Here's how the part is built. I have some questions about the finished solid (model axes, mm). Coordinates: 2 decimals unless noted, no trailing zeros. Write each loop counter-clockwise with the first axis right and the second up, starting at its lowest first coordinate (ties: lowest second). Pieces come first, ordered by that corner, then holes.
Item 1: If we section it at A-A (x = 0): Please give me the cut outline in (y, z) (3 decimals), then the cut area to 3 significant figures.
Item 2: If we section it at B-B (y = -128): Please give me the cut outline in (x, z) (3 decimals).
Item 3: I'm going to push flat-ended pins straight in: pin 1 Ø4 at (y, z) = (-240, -18) entering from +X; pin 2 Ø11.5 at (x, z) = (0, 0) entering from +Y; pin 3 Ø1.5 at (y, z) = (-148, 9.5) entering from -X. Where does each tip first touch, or does it pass through?
Item 4: If I drill on line 1 (Y direction, x = -9, z = 13); line 2 (Z direction, x = 0, y = -126) (3 decimals), over which ranges is the centre line in solid material (lowest first)?
Item 5: If we section it at C-C (z = 0): Please give me the cut outline in (x, y) (3 decimals).
from build123d import *

# Parameters (mm, degrees)
F0_R          = 34.925
F0_R_2        = 28.575
F1_DEPTH      = 304.8
F2_R          = 34.925
F3_DEPTH      = 6.35
F4_R          = 34.925
F5_DEPTH      = 6.35
F6_R          = 6.35
F7_R          = 6.35
F8_W          = 228.6
F8_H          = 3.175
F10_S5_R      = 34.925
F10_T6_DEPTH  = 52
F10_S11_R     = 31.75
F10_T12_DEPTH = 51
F11_R         = 6.35
F12_DEPTH     = 25.4


# Not quite as in the source:
# - a fillet or chamfer that OpenCascade refuses, or shapes differently, is made with other operations: its cross-section is extruded or revolved along the edge and cut away or added


with BuildPart() as f1:
    # F0 (on Front) → F1 (new body)
    with BuildSketch(Plane.XZ):
        Circle(F0_R)
        Circle(F0_R_2, mode=Mode.SUBTRACT)
    extrude(amount=F1_DEPTH)

    # F2 (on face) → F3 (join)
    with BuildSketch(Plane.XZ.offset(304.8)):
        Circle(F2_R)
    extrude(amount=-F3_DEPTH)

    # F4 (on face) → F5 (join)
    with BuildSketch(Plane(origin=(0, 0, 0), x_dir=(-1, 0, 0), z_dir=(0, 1, 0))):
        Circle(F4_R)
    extrude(amount=-F5_DEPTH)

    # F6
    f6_edges = [f1.edges().sort_by_distance(p)[0] for p in [
        (-34.925, 0, 0),
    ]]
    fillet(f6_edges, radius=F6_R)

    # F7
    f7_edges = [f1.edges().sort_by_distance(p)[0] for p in [
        (-34.925, -304.8, 0),
    ]]
    fillet(f7_edges, radius=F7_R)

    # F8 (on Right) → F9 (revolve, cut)
    with BuildSketch(Plane.YZ):
        with Locations((-152.4, -33.3375)):
            Rectangle(F8_W, F8_H)
    revolve(axis=Axis((0, -304.8, 0), (0, -1, 0)), mode=Mode.SUBTRACT)

    # F10: chamfer of 10.16 x 3.6979375801 on 2 edges, made by hand


with BuildPart() as f10_tool2:
    # F10_s3 → F10_t4 (revolve)
    with BuildSketch(Plane.YZ):
        Polygon((-48.26, -31.75), (-38.1, -35.4479375801), (-38.1, -31.75), align=None)
    revolve(axis=Axis((0, -38.1, 0), (0, -1, 0)))

    # F10_s5 → F10_t6 (intersect, symmetric)
    with BuildSketch(Plane.XZ.offset(43.2)):
        Circle(F10_S5_R)
    extrude(amount=F10_T6_DEPTH, both=True, mode=Mode.INTERSECT)


with BuildPart() as f1_1:
    add(f1.part)

    # F10_t1: union F10_tool2
    add(f10_tool2.part)


with BuildPart() as f10_tool8:
    # F10_s9 → F10_t10 (revolve)
    with BuildSketch(Plane.XY):
        Polygon((34.925, -276.86), (31.2270624199, -266.7), (34.925, -266.7), align=None)
    revolve(axis=Axis((0, -266.7, 0), (0, -1, 0)))

    # F10_s11 → F10_t12 (cut, symmetric)
    with BuildSketch(Plane.XZ.offset(271.8)):
        Circle(F10_S11_R)
    extrude(amount=F10_T12_DEPTH, both=True, mode=Mode.SUBTRACT)


with BuildPart() as f1_2:
    add(f1_1.part)

    # F10_t7: cut F10_tool8
    add(f10_tool8.part, mode=Mode.SUBTRACT)

    # F11 (on face) → F12 (cut)
    with BuildSketch(Plane(origin=(0, 0, 0), x_dir=(-1, 0, 0), z_dir=(0, 1, 0))):
        Circle(F11_R)
    extrude(amount=-F12_DEPTH, mode=Mode.SUBTRACT)


solid = f1_2.part
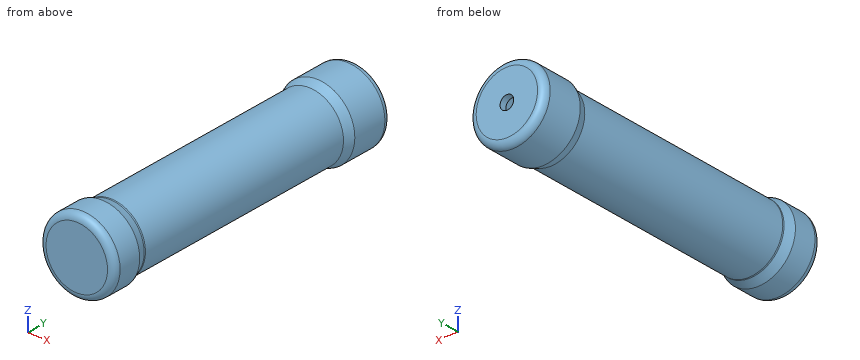
Answer list:
1. outline: (-304.8, -28.575) arc R6.35 ccw to (-298.45, -34.925) - (-276.86, -34.925) - (-268.137, -31.75) - (-48.26, -31.75) - (-39.537, -34.925) - (-6.35, -34.925) arc R6.35 ccw to (0, -28.575) - (0, -6.35) - (-6.35, -6.35) - (-6.35, -28.575) - (-298.45, -28.575) - (-298.45, 28.575) - (-6.35, 28.575) - (-6.35, 6.35) - (0, 6.35) - (0, 28.575) arc R6.35 ccw to (-6.35, 34.925) - (-39.537, 34.925) - (-48.26, 31.75) - (-268.137, 31.75) - (-276.86, 34.925) - (-298.45, 34.925) arc R6.35 ccw to (-304.8, 28.575) - close
1. area: 3,030 mm2
2. outline: circle Ø63.5 at (0, 0); hole circle Ø57.15 at (0, 0)
3. pin 1: stops at x = 27.42
3. pin 2: stops at y = -298.45
3. pin 3: stops at x = -30.52
4. line 1: y = -304.8 to -298.45, -6.35 to 0
4. line 2: z = -31.75 to -28.575, 28.575 to 31.75
5. outline: (-34.925, -298.45) arc R6.35 ccw to (-28.575, -304.8) - (28.575, -304.8) arc R6.35 ccw to (34.925, -298.45) - (34.925, -276.86) - (31.75, -268.137) - (31.75, -48.26) - (34.925, -39.537) - (34.925, -6.35) arc R6.35 ccw to (28.575, 0) - (6.35, 0) - (6.35, -6.35) - (28.575, -6.35) - (28.575, -298.45) - (-28.575, -298.45) - (-28.575, -6.35) - (-6.35, -6.35) - (-6.35, 0) - (-28.575, 0) arc R6.35 ccw to (-34.925, -6.35) - (-34.925, -39.537) - (-31.75, -48.26) - (-31.75, -268.137) - (-34.925, -276.86) - close
